Here's how the part is built. I have some questions about the finished solid (model axes, mm). A direction names the side the tool comes from. Round coordinates to 2 decimals unless told otherwise and drop trailing zeros. Order: outer loops, then holes, each group sorted by start corner. A loop starts at its lowest first (then second) coordinate and runs counter-clockwise, first axis right, second up. Notation, with made-up numbers: (26, -36.75) -> (30, -36.75) arc R26 ccw to (30, -0.75) -> close; hole circle Ø5 at (79.25, 53.25). An arc over 180 degrees is marked (long way). Use a Markdown table: item, result. Add a question column.
(1) Thinking about a two-plate mould opening in Z: for faces 4 (the face through (64.06, 5.92, 20.58)), 5 (the face through (-60, 6, -31)), 6 (the face through (0, 24, -40)), 7 (the face through (6, 41, 9)), which applies, pulls with the +Z half, pulls with the -Z half, needs draft (parallel to the pull), parting line crosses it, or undercut?
(2) I want a section at B-B, the plane y = 54.5. Please give me the cut outline in (x, z).
(3) I want a section at D-D, the plane x = 0. Please give me the cut outline in (y, z), then the cut area to 3 significant figures.
(4) On a 3-axis mill with a long thin cutter (end or side, diameter ignored), from which of +Z, -Z, +X, -X, +Y, -Y can I reach the whole of each face in a straight line? I mean faces 1 (the face through (40, 12, -1)), 2 (the face through (-6, 41, 9)), 3 (the face through (0, 24, 40)). Say none if no direction works.
(5) If I drill on probe 1 along X at (y, z) = (8.5, 25); probe 2 along Z at (x, y) = (1, 54); probe 3 along Y at (x, z) = (48.5, 14), over which ranges is the centre line in solid material (lowest first)?
(6) I want a section at C-C, the plane z = 0. Please give me the cut outline in (x, y).
(7) I'm going to push flat-ended pins straight in: P1, Ø19, axis at x = -60, z = 25, coming from the +Y side; P2, Ø12, axis at y = 63.5, z = -22.5, coming from the +X side; P3, Ø3, axis at x = -33, z = -0.5, coming from the -Y side; P4, Ø22.5, axis at y = 63, z = 7, coming from the -X side. Where does each tip first touch, or does it pass through?
(8) I want a section at A-A, the plane x = -60. Please give me the cut outline in (y, z).
from build123d import *

# Parameters (mm, degrees)
ESBO_O1_W                = 150
ESBO_O1_H                = 80
ESBO_O1_R                = 6
RESSALTO_EXTRUS_O1_DEPTH = 12
ESBO_O2_W                = 12
ESBO_O2_H                = 80
RESSALTO_EXTRUS_O2_DEPTH = 75
ESBO_O3_R                = 16
CORTE_EXTRUS_O1_DEPTH    = 126.419296761


with BuildPart() as part:
    # Esboço1 → Ressalto-extrusão1 (new body)
    with BuildSketch(Plane(origin=(0, 0, 0), x_dir=(1, 0, 0), z_dir=(0, 1, 0))):
        Rectangle(ESBO_O1_W, ESBO_O1_H)
        with Locations(Location((-60, 25, 0), (0, 0, 270))):
            Circle(ESBO_O1_R, mode=Mode.SUBTRACT)
        with Locations(Location((-60, -25, 0), (0, 0, 270))):
            Circle(ESBO_O1_R, mode=Mode.SUBTRACT)
        with Locations(Location((60, 25, 0), (0, 0, 270))):
            Circle(ESBO_O1_R, mode=Mode.SUBTRACT)
        with Locations(Location((60, -25, 0), (0, 0, 270))):
            Circle(ESBO_O1_R, mode=Mode.SUBTRACT)
    extrude(amount=RESSALTO_EXTRUS_O1_DEPTH)

    # Esboço2 → Ressalto-extrusão2 (add)
    with BuildSketch(Plane(origin=(0, 12, 0), x_dir=(1, 0, 0), z_dir=(0, 1, 0))):
        Rectangle(ESBO_O2_W, ESBO_O2_H)
    extrude(amount=RESSALTO_EXTRUS_O2_DEPTH)

    # Esboço3 → Corte-extrusão1 (cut, through all)
    with BuildSketch(Plane.ZY.offset(6)):
        with Locations((0, 54.5)):
            Circle(ESBO_O3_R)
    extrude(amount=-CORTE_EXTRUS_O1_DEPTH, mode=Mode.SUBTRACT)


solid = part.part
Taken from the geometry:
| question | item | result |
|---|---|---|
| 1 | face 4 | undercut |
| 1 | face 5 | undercut |
| 1 | face 6 | pulls with the -Z half |
| 1 | face 7 | needs draft |
| 2 | outline | (-6, -40) -> (6, -40) -> (6, -16) -> (-6, -16) -> close; (-6, 16) -> (6, 16) -> (6, 40) -> (-6, 40) -> close |
| 3 | outline | (0, -40) -> (87, -40) -> (87, 40) -> (0, 40) -> close; hole circle Ø32 at (54.5, 0) |
| 3 | area | 6,160 mm2 |
| 4 | face 1 | +Z, -Z, +X, +Y |
| 4 | face 2 | +Z, -Z, -X, +Y |
| 4 | face 3 | +Z, +X, -X, +Y, -Y |
| 5 | probe 1 | x = -75 to -66, -54 to 54, 66 to 75 |
| 5 | probe 2 | z = -40 to -15.99, 15.99 to 40 |
| 5 | probe 3 | y = 0 to 12 |
| 6 | outline | (-75, 0) -> (75, 0) -> (75, 12) -> (6, 12) -> (6, 38.5) -> (-6, 38.5) -> (-6, 12) -> (-75, 12) -> close; (-6, 70.5) -> (6, 70.5) -> (6, 87) -> (-6, 87) -> close |
| 7 | P1 | stops at y = 12 |
| 7 | P2 | stops at x = 6 |
| 7 | P3 | stops at y = 0 |
| 7 | P4 | stops at x = -6 |
| 8 | outline | (0, -40) -> (12, -40) -> (12, -31) -> (0, -31) -> close; (0, -19) -> (12, -19) -> (12, 19) -> (0, 19) -> close; (0, 31) -> (12, 31) -> (12, 40) -> (0, 40) -> close |
